Read the model definition and answer for the solid it produces. Units are mm, in the model's axes. A direction names the side the tool comes from. Coordinates: 2 decimals unless noted, no trailing zeros. Write each loop counter-clockwise with the first axis right and the second up, starting at its lowest first coordinate (ties: lowest second). Pieces come first, ordered by that corner, then holes.
(1) Which of the six approach directions +Z, -Z, +X, -X, +Y, -Y give full straight-line access (tool end or side, diameter ignored) to faces 4 (the flat face through (6, 0, 265)), 5 (the flat face through (0, 0, 0)), 6 (the cylindrical face through (2.7, -2.4, 4.9))?
(2) The mould has two halves that part along X. Classify faces 1 (the cylindrical face through (2.7, -2.4, 270.1)), 2 (the flat face through (15, -4.5, 135.6)), 3 (the flat face through (-3, -7, 136)): +X half, -X half, draft (parallel to the pull), parting line (faces both ways), or undercut.
(3) Section B-B on z = 222 is taken. Write down the section's boundary in (x, y).
(4) Find the intervals of material crossed by probe 1 along Y at (x, z) = (5.9, 271.5); probe 2 along Y at (x, z) = (5, 2); probe 3 along Y at (x, z) = (15, 183.5), in increasing order.
(5) Section A-A on x = 5.9 is taken. Write down the section's boundary in (y, z), then the cut area to 3 significant figures.
(6) Given pin 1 (5 mm diameter, centred on x = 5.9, y = 0, fed in from +Z); pin 2 (4 mm diameter, centred on x = 11, y = 3, fed in from -Z); pin 3 (1.5 mm diameter, centred on y = -4.5, z = 101, fed in from +X), each flat-ended and moving along its own axis, determine where each tip first touches the part or whether it passes through.
from build123d import *

# Parameters (mm, degrees)
SKETCH_1_W          = 35
SKETCH_1_H          = 14
EXTRUDE_1_DEPTH     = 275
CHAMFER_1_SIZE      = 5
SKETCH_2_R          = 4
CUT_EXTRUDE_1_DEPTH = 10


with BuildPart() as part:
    # 草图1 → 凸台-拉伸1 (new body)
    with BuildSketch(Plane.XY):
        Rectangle(SKETCH_1_W, SKETCH_1_H)
    extrude(amount=EXTRUDE_1_DEPTH)

    # 倒角1
    chamfer_1_edges = [part.edges().sort_by_distance(p)[0] for p in [
        (17.5, -7, 137.5),
    ]]
    chamfer(chamfer_1_edges, length=CHAMFER_1_SIZE)

    # 草图2 → 切除-拉伸1 (cut)
    with BuildSketch(Plane.XY.offset(275)):
        with Locations((5.9, 0)):
            Circle(SKETCH_2_R)
    cut_extrude_1 = extrude(amount=-CUT_EXTRUDE_1_DEPTH, mode=Mode.SUBTRACT)

    # 镜向1: 切除-拉伸1 across plane
    add(cut_extrude_1.mirror(Plane(origin=(0, 0, 137.5), x_dir=(1, 0, 0), z_dir=(0, 0, -1))), mode=Mode.SUBTRACT)


solid = part.part
Response:
1. face 4: +Z
1. face 5: -Z, +X, -X, +Y, -Y
1. face 6: -Z
2. face 1: undercut
2. face 2: +X half
2. face 3: draft
3. outline: (-17.5, -7) - (12.5, -7) - (17.5, -2) - (17.5, 7) - (-17.5, 7) - close
4. probe 1: y = -7 to -4, 4 to 7
4. probe 2: y = -7 to -3.9, 3.9 to 7
4. probe 3: y = -4.5 to 7
5. outline: (-7, 0) - (-4, 0) - (-4, 10) - (4, 10) - (4, 0) - (7, 0) - (7, 275) - (4, 275) - (4, 265) - (-4, 265) - (-4, 275) - (-7, 275) - close
5. area: 3,690 mm2
6. pin 1: stops at z = 265
6. pin 2: stops at z = 0
6. pin 3: stops at x = 15.75
